Job drawing, mm, ordinate dimensions from the low corner. One solid piece. Give positions to 0.01 mm unless a question says otherwise; leave off trailing zeros. Order: outer loops, then holes, each group sorted by start corner. A loop starts at its lowest first (then second) coordinate and runs counter-clockwise, first axis right, second up. Notation, with made-up numbers: M -21,19 L 30,19 A12 cw 30,39 Z; hole C -29,17.5 d3. An arc over 180 degrees is marked long. Put each result on its own line as item: value. Start each with the question number.
1) Drill centre lines: line 1 (Y direction, x = 12.7, z = 0.75); line 2 (X direction, y = 14.25, z = 1.4); line 3 (Y direction, x = 266, z = 1.65). Where is each one in solid material? Low to high. Write a range as [from, to].
2) Cut at B-B (x = 12.7). Write the cut outline in (y, z).
3) Cut at A-A (y = 12.7). Write the cut outline in (x, z).
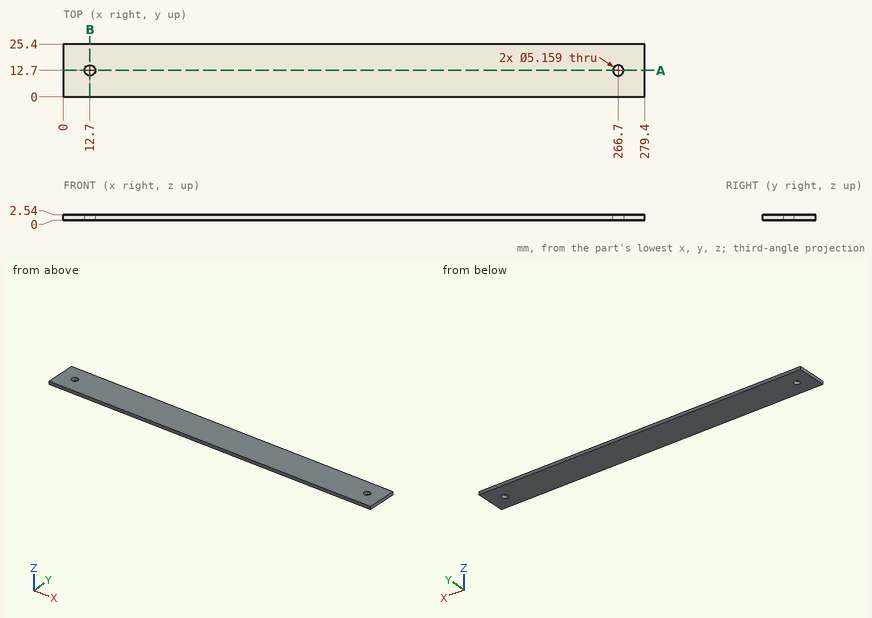
Solution:
1. line 1: [0, 10.12], [15.28, 25.4]
1. line 2: [0, 10.64], [14.76, 264.64], [268.76, 279.4]
1. line 3: [0, 10.22], [15.18, 25.4]
2. outline: M 0,0 L 10.12,0 L 10.12,2.54 L 0,2.54 Z; M 15.28,0 L 25.4,0 L 25.4,2.54 L 15.28,2.54 Z
3. outline: M 0,0 L 10.12,0 L 10.12,2.54 L 0,2.54 Z; M 15.28,0 L 264.12,0 L 264.12,2.54 L 15.28,2.54 Z; M 269.28,0 L 279.4,0 L 279.4,2.54 L 269.28,2.54 Z
